from build123d import *

# Parameters (mm, degrees)
F0_W        = 88.9
F0_H        = 57.15
F1_DEPTH    = 3.81
F2_W        = 6.35
F2_H        = 57.15
F3_DEPTH    = 7.62
F4_W        = 95.25
F4_H        = 6.35
F5_DEPTH    = 7.62
F6_W        = 6.35
F6_H        = 63.5
F7_DEPTH    = 7.62
F8_W        = 101.6
F8_H        = 6.35
F9_DEPTH    = 7.62
F9_FACE_W   = 101.6
F9_FACE_H   = 69.85
F9_FACE_W_2 = 88.9
F9_FACE_H_2 = 57.15
F10_DEPTH   = 12.7


with BuildPart() as f1:
    # F0 (on Top) → F1 (new body)
    with BuildSketch(Plane.XY):
        Rectangle(F0_W, F0_H)
    extrude(amount=F1_DEPTH)

    # F2 (on Top) → F3 (join)
    with BuildSketch(Plane.XY):
        with Locations((-47.625, 0)):
            Rectangle(F2_W, F2_H)
    extrude(amount=F3_DEPTH)

    # F4 (on Top) → F5 (join)
    with BuildSketch(Plane.XY):
        with Locations((-3.175, -31.75)):
            Rectangle(F4_W, F4_H)
    extrude(amount=F5_DEPTH)

    # F6 (on Top) → F7 (join)
    with BuildSketch(Plane.XY):
        with Locations((47.625, -3.175)):
            Rectangle(F6_W, F6_H)
    extrude(amount=F7_DEPTH)

    # F8 (on Top) → F9 (join)
    with BuildSketch(Plane.XY):
        with Locations((0, 31.75)):
            Rectangle(F8_W, F8_H)
    extrude(amount=F9_DEPTH)

    # F9_face (on face) → F10 (join)
    with BuildSketch(Plane.XY.offset(7.62)):
        Rectangle(F9_FACE_W, F9_FACE_H)
        Rectangle(F9_FACE_W_2, F9_FACE_H_2, mode=Mode.SUBTRACT)
    extrude(amount=F10_DEPTH)


solid = f1.part
Verification items for the finished model (mm, model axes). A direction names the side the tool comes from. Give positions to 0.01 mm unless a question says otherwise; leave off trailing zeros. Write each loop counter-clockwise with the first axis right and the second up, starting at its lowest first coordinate (ties: lowest second). Pieces come first, ordered by that corner, then holes. Notation, with made-up numbers: (-1.5, 60.5) -> (13.5, 60.5) arc R8 ccw to (13.5, 65.5) -> close; hole circle Ø10 at (74, -26). An arc over 180 degrees is marked (long way). Use CSV: the item, a comma, the result in double quotes.
(1) Release check for a two-part mould opening along X. For faces 1 (the flat face through (50.8, 0, 10)), 2 (the flat face through (-1, -28.575, 12)), 3 (the flat face through (-1, -34.925, 10)), 4 (the flat face through (-50.8, 0, 10)) record: +X half, -X half, draft (parallel to the pull), parting line (faces both ways), or undercut.
Derived:
face 1,"+X half"
face 2,"undercut"
face 3,"draft"
face 4,"-X half"
(2) Set-up check for faces 5 (the flat face through (-1, 0, 3.81)), 6 (the flat face through (-1, 0, 0)): record each of +Z, -Z, +X, -X, +Y, -Y from which the full face is reachable in a straight line by a thin tool's end or side.
Derived:
face 5,"+Z"
face 6,"-Z, +X, -X, +Y, -Y"
(3) Go/stop test with flat-tipped pins: pin 1 (3 mm diameter, centred on x = -40, y = 17, fed in from +Z); pin 2 (3 mm diameter, centred on x = 11, y = -17, fed in from -Z). Record where each tip stops, or that it passes through.
Derived:
pin 1,"stops at z = 3.81"
pin 2,"stops at z = 0"
(4) Sectioned sample at A-A (x = 11). Record the cut outline in (y, z) (3 decimals), plus the area to 3 significant figures.
Derived:
outline,"(-34.925, 0) -> (34.925, 0) -> (34.925, 20.32) -> (28.575, 20.32) -> (28.575, 3.81) -> (-28.575, 3.81) -> (-28.575, 20.32) -> (-34.925, 20.32) -> close"
area,"476 mm^2"
(5) Material ranges on L1, parallel to X at y = 23, z = 14.5; L2, parallel to Y at x = -35.5, z = 14.5 (3 decimals); L3, parallel to Z at x = -5, y = 5, recorded low to high.
Derived:
L1,"x = -50.8 to -44.45, 44.45 to 50.8"
L2,"y = -34.925 to -28.575, 28.575 to 34.925"
L3,"z = 0 to 3.81"
(6) Sectioned sample at B-B (z = 17.5). Record the cut outline in (x, y) (3 decimals), plus the area to 3 significant figures.
Derived:
outline,"(-50.8, -34.925) -> (50.8, -34.925) -> (50.8, 34.925) -> (-50.8, 34.925) -> close; hole (-44.45, -28.575) -> (44.45, -28.575) -> (44.45, 28.575) -> (-44.45, 28.575) -> close"
area,"2,020 mm^2"
(7) Sectioned sample at C-C (y = -10.5). Record the cut outline in (x, z), plus the area to 3 significant figures.
Derived:
outline,"(-50.8, 0) -> (50.8, 0) -> (50.8, 20.32) -> (44.45, 20.32) -> (44.45, 3.81) -> (-44.45, 3.81) -> (-44.45, 20.32) -> (-50.8, 20.32) -> close"
area,"597 mm^2"
